Autodesk Inventor part; units mm, degrees
ref_plane "p1_XY" through (0, 0, 0) normal (1, 0, 0) x (0, 0, -1)
ref_plane "p1_YZ" through (0, 0, 0) normal (0, 0, -1) x (0, 1, 0)
ref_plane "p1_ZX" through (0, 0, 0) normal (0, 1, 0) x (1, 0, 0)
sketch "Sketch_1" plane through (0, 0, 0) normal (0, 0, 1) x (1, 0, 0)
  line L0 (50, 0) -> (-50, 0)
  line L1 (-13.5, 0) -> (-13.5, 2)
  line L2 (-13.5, 2) -> (-6.75, 2)
  line L3 (-6.75, 2) -> (-6.75, 13.5)
  line L4 (-6.75, 13.5) -> (6.75, 13.5)
  line L5 (6.75, 13.5) -> (6.75, 2)
  line L6 (6.75, 2) -> (13.5, 2)
  line L7 (13.5, 2) -> (13.5, 0)
  line L8 (13.5, 0) -> (-13.5, 0)
revolve "Revolution1" add sketch "Sketch_1" angle 360 about axis through (50, 0, 0) along (1, 0, 0)
ref_plane "p1_XY" through (0, 0, 0) normal (1, 0, 0) x (0, 0, -1)
ref_plane "p1_YZ" through (0, 0, 0) normal (0, 0, -1) x (0, 1, 0)
ref_plane "p1_ZX" through (0, 0, 0) normal (0, 1, 0) x (1, 0, 0)
properties part number "PRO10314 Rollenleiste Grundteil"
Geometry check sheet. Reference: the model listing, model coordinates, mm. A direction names the side the tool comes from. Give positions to 0.01 mm unless a question says otherwise; leave off trailing zeros. Write each loop counter-clockwise with the first axis right and the second up, starting at its lowest first coordinate (ties: lowest second). Pieces come first, ordered by that corner, then holes. Notation, with made-up numbers: (42, 46.5) - (48, 46.5) arc R31 cw to (48, 84.5) - close; hole circle Ø3 at (19.25, -28). An arc over 180 degrees is marked (long way). Put each result on its own line as item: value.
1. Thickness scan on line 1 (X direction, y = 9.25, z = -7.5); line 2 (Z direction, x = -1, y = 10.75); line 3 (Y direction, x = -5, z = -1.5). Record the ranges inside material, lowest first.
Ans:
line 1: x = -6.75 to 6.75
line 2: z = -8.17 to 8.17
line 3: y = -13.42 to 13.42
2. Set-up check for faces 1 (the cylindrical face through (0.09, -2.93, -13.18)), 2 (the cylindrical face through (-10, 0, -2)), 3 (the cylindrical face through (10, 0, -2)): record each of +Z, -Z, +X, -X, +Y, -Y from which the full face is reachable in a straight line by a thin tool's end or side.
Ans:
face 1: +X, -X
face 2: -X
face 3: +X
3. Go/stop test with flat-tipped pins: pin 1 (3 mm diameter, centred on y = -4.5, z = -9, fed in from -X); pin 2 (5 mm diameter, centred on x = -5, y = 6.5, fed in from +Z); pin 3 (3 mm diameter, centred on x = -2.5, y = -10, fed in from -Z). Record where each tip stops, or that it passes through.
Ans:
pin 1: stops at x = -6.75
pin 2: stops at z = 12.89
pin 3: stops at z = -10.49
4. Sectioned sample at D-D, the plane x = -3.5. Enter the section's corners in (y, z), plus the area to 3 significant figures.
Ans:
outline: circle Ø27 at (0, 0)
area: 573 mm²
5. Sectioned sample at C-C, the plane x = -9. Enter the section's corners in (y, z).
Ans:
outline: circle Ø4 at (0, 0)
6. Sectioned sample at A-A, the plane z = 0. Enter the section's corners in (x, y).
Ans:
outline: (-13.5, -2) - (-6.75, -2) - (-6.75, -13.5) - (6.75, -13.5) - (6.75, -2) - (13.5, -2) - (13.5, 2) - (6.75, 2) - (6.75, 13.5) - (-6.75, 13.5) - (-6.75, 2) - (-13.5, 2) - close
